Answer from the drawing. Dimensions are ordinates in mm from the lowest x, y and z of the part. A direction names the side the tool comes from. Round coordinates to 2 decimals unless told otherwise and drop trailing zeros. Order: outer loops, then holes, each group sorted by start corner. A loop starts at its lowest first (then second) coordinate and runs counter-clockwise, first axis right, second up. Notation, with made-up numbers: (24, 56.25) -> (32, 56.25) arc R29 cw to (32, 93.25) -> close; hole circle Ø9 at (24, -37). An arc over 180 degrees is marked (long way). Use a Markdown table: item, result. Add a question column.
Item 1: A cutting plane is placed at D-D, the plane z = 5. Determine the outline of the cut face in (x, y).
Item 2: A cutting plane is placed at C-C, the plane z = 12.5. Determine the outline of the cut face in (x, y).
Item 3: A cutting plane is placed at A-A, the plane x = 8. Determine the outline of the cut face in (y, z), plus the area to 3 significant figures.
Item 4: Find the intervals of material crossed by L1, parallel to Z at x = 1, y = 17; L2, parallel to Z at x = 26, y = 2.1; L3, parallel to X at y = 11.5, z = 11.5, in increasing order. Write a range as [from, to].
Item 5: A cutting plane is placed at B-B, the plane y = 17. Determine the outline of the cut face in (x, z), plus the area to 3 significant figures.
Item 6: Flat-ended cylindrical pins translate along their axes: P1, Ø12, axis at x = 14.5, y = 18.5, coming from the +Z side; P2, Ø5, axis at y = 17, z = 21, coming from the +X side; P3, Ø6, axis at x = 26, z = 20, coming from the +Y side. Find the tip coordinate at first contact, or state that the pin passes through.
Item 7: A tool of negligible diameter and unlimited length cuts with its end or side. For the marked faces 1 and 2, from which of +Z, -Z, +X, -X, +Y, -Y can it reach the whole face along a straight path? Write none if from no direction.
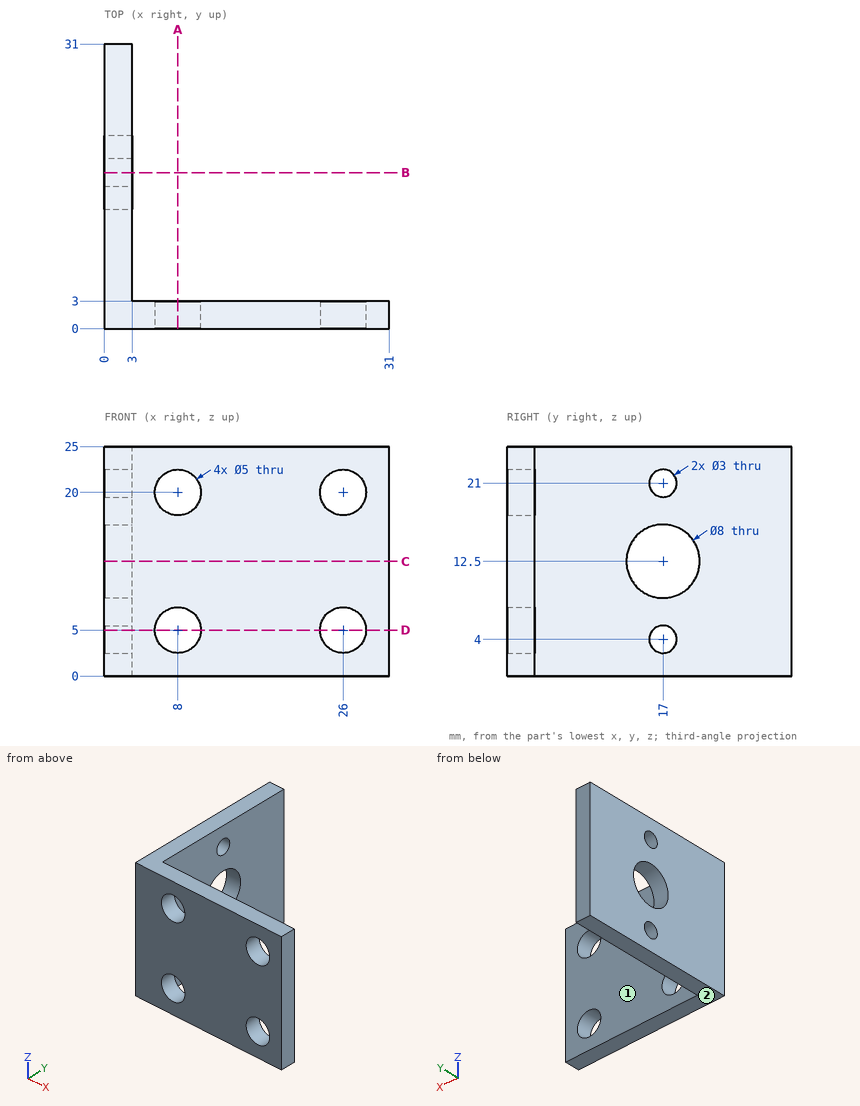
Reported:
| question | item | result |
|---|---|---|
| 1 | outline | (0, 0) -> (5.5, 0) -> (5.5, 3) -> (3, 3) -> (3, 15.88) -> (0, 15.88) -> close; (0, 18.12) -> (3, 18.12) -> (3, 31) -> (0, 31) -> close; (10.5, 0) -> (23.5, 0) -> (23.5, 3) -> (10.5, 3) -> close; (28.5, 0) -> (31, 0) -> (31, 3) -> (28.5, 3) -> close |
| 2 | outline | (0, 0) -> (31, 0) -> (31, 3) -> (3, 3) -> (3, 13) -> (0, 13) -> close; (0, 21) -> (3, 21) -> (3, 31) -> (0, 31) -> close |
| 3 | outline | (0, 0) -> (3, 0) -> (3, 2.5) -> (0, 2.5) -> close; (0, 7.5) -> (3, 7.5) -> (3, 17.5) -> (0, 17.5) -> close; (0, 22.5) -> (3, 22.5) -> (3, 25) -> (0, 25) -> close |
| 3 | area | 45.0 mm² |
| 4 | L1 | [0, 2.5], [5.5, 8.5], [16.5, 19.5], [22.5, 25] |
| 4 | L2 | [0, 2.5], [7.5, 17.5], [22.5, 25] |
| 4 | L3 | [0, 3] |
| 5 | outline | (0, 0) -> (3, 0) -> (3, 2.5) -> (0, 2.5) -> close; (0, 5.5) -> (3, 5.5) -> (3, 8.5) -> (0, 8.5) -> close; (0, 16.5) -> (3, 16.5) -> (3, 19.5) -> (0, 19.5) -> close; (0, 22.5) -> (3, 22.5) -> (3, 25) -> (0, 25) -> close |
| 5 | area | 33.0 mm² |
| 6 | P1 | through |
| 6 | P2 | x = 3 |
| 6 | P3 | y = 3 |
| 7 | face 1 | +Z, -Z, +X, +Y |
| 7 | face 2 | -Z, +X, -X, +Y, -Y |
